Work out the finished part from the listing and answer in its coordinate system (mm). A direction names the side the tool comes from. Round coordinates to 2 decimals unless told otherwise and drop trailing zeros. Loops run counter-clockwise (first coordinate to the right, second up) from the corner with the lowest first, then second, coordinate; pieces in that order, holes last. Notation, with made-up numbers: M 6,-9.75 L 23,-9.75 A17 ccw 23,16.25 Z; hole C 46.5,44 d8. An arc over 180 degrees is marked long. One line per item, written item: value.
```python
from build123d import *

# Parameters (mm, degrees)
F0_W     = 101.6
F0_H     = 50.8
F1_DEPTH = 25.4
F2_R     = 6.35
F3_DEPTH = 12.7
F6_SIZE  = 2.54


with BuildPart() as f1:
    # F0 (on Front) → F1 (new body)
    with BuildSketch(Plane.XZ):
        Rectangle(F0_W, F0_H)
    extrude(amount=F1_DEPTH)

    # F2 (on face) → F3 (cut)
    with BuildSketch(Plane(origin=(0, 0, 0), x_dir=(-1, 0, 0), z_dir=(0, 1, 0))):
        with Locations((31.75, -12.7)):
            Circle(F2_R)
        with Locations((-31.75, 12.7)):
            Circle(F2_R)
        with Locations((-31.75, -12.7)):
            Circle(F2_R)
        with Locations((31.75, 12.7)):
            Circle(F2_R)
    extrude(amount=-F3_DEPTH, mode=Mode.SUBTRACT)

    # F4 (on Top) → F5 (revolve)
    with BuildSketch(Plane.XY):
        Polygon((-16.995588, 0), (0, 0), (0, 42.096764), (-16.995588, 42.096764), (-16.995588, 27.715884), (-12.550589, 27.715884), (-12.550589, 16.734118), (-16.995588, 16.734118), align=None)
    revolve(axis=Axis((0, 21.048382, 0), (0, 1, 0)))

    # F6
    f6_edges = [f1.edges().sort_by_distance(p)[0] for p in [
        (16.995588, 16.734118, 0),
        (16.995588, 27.715884, 0),
    ]]
    chamfer(f6_edges, length=F6_SIZE)


solid = f1.part
```
1) Each of these flat-tipped pins is pushed along its axis until it touches: pin 1 (14 mm diameter, centred on x = 33.5, z = -9.5, fed in from +Y); pin 2 (5 mm diameter, centred on y = 28.5, z = 12.5, fed in from +X); pin 3 (7.5 mm diameter, centred on x = 31.75, z = -12.7, fed in from +Y). Where does it stop, or does it pass through?
Check values:
pin 1: y = 0
pin 2: x = 13.19
pin 3: y = -12.7
2) Find section D-D (x = -21). Give the vertices of the cut face in (y, z).
Check values:
outline: M -25.4,-25.4 L 0,-25.4 L 0,25.4 L -25.4,25.4 Z
3) Find section B-B (x = 31.75). Give the vertices of the cut face in (y, z), then the cut area to 3 significant figures.
Check values:
outline: M -25.4,-25.4 L 0,-25.4 L 0,-19.05 L -12.7,-19.05 L -12.7,-6.35 L 0,-6.35 L 0,6.35 L -12.7,6.35 L -12.7,19.05 L 0,19.05 L 0,25.4 L -25.4,25.4 Z
area: 968 mm2
4) Find section A-A (x = 0). Give the vertices of the cut face in (y, z).
Check values:
outline: M -25.4,-25.4 L 0,-25.4 L 0,-17 L 14.19,-17 L 16.73,-14.46 L 16.73,-12.55 L 27.72,-12.55 L 27.72,-14.46 L 30.26,-17 L 42.1,-17 L 42.1,17 L 30.26,17 L 27.72,14.46 L 27.72,12.55 L 16.73,12.55 L 16.73,14.46 L 14.19,17 L 0,17 L 0,25.4 L -25.4,25.4 Z
5) For faces 4 (the face through (0, 27.716, 13)), 5 (the face through (-1, -13, -25.4)), 6 (the face through (-16.21, 36.09, 5.11)), determine the directions among +Z, -Z, +X, -X, +Y, -Y from which every point of the face is accessible in a straight line to the end or side of a thin tool.
Check values:
face 4: none
face 5: -Z, +X, -X, +Y, -Y
face 6: +Y
6) Find the intervals of material crossed by probe 1 along Z at (x, y) = (-31.75, -6.75); probe 2 along Y at (x, z) = (0.5, -14); probe 3 along X at (y, z) = (-3, 12), in increasing order. Write a range as from..to.
Check values:
probe 1: -25.4..-19.05, -6.35..6.35, 19.05..25.4
probe 2: -25.4..16.73, 27.72..42.1
probe 3: -50.8..-38.06, -25.44..25.44, 38.06..50.8
7) The mould has two halves that part along Y. Classify faces 1 (the face through (-13.94, 27.875, 4.39)), 2 (the face through (-1, -13, 25.4)), 3 (the face through (-32, -12.7, 13)): +Y half, -Y half, draft (parallel to the pull), parting line (faces both ways), or undercut.
Check values:
face 1: undercut
face 2: draft
face 3: +Y half
8) Find section C-C (x = -36). Give the vertices of the cut face in (y, z).
Check values:
outline: M -25.4,-25.4 L 0,-25.4 L 0,-17.42 L -12.7,-17.42 L -12.7,-7.98 L 0,-7.98 L 0,7.98 L -12.7,7.98 L -12.7,17.42 L 0,17.42 L 0,25.4 L -25.4,25.4 Z
